Source: CAD feature listing. Evaluate the final solid. Frame: model axes, mm. A direction names the side the tool comes from. Give positions to 0.01 mm unless a question says otherwise; leave off trailing zeros. Loops run counter-clockwise (first coordinate to the right, second up) from the corner with the lowest first, then second, coordinate; pieces in that order, holes last. Notation, with made-up numbers: M 21.25,5.25 L 40.25,5.25 A17 ccw 40.25,33.25 Z; hole C 14.25,32.5 d11. An arc over 180 degrees is marked long. Answer in a Markdown table with one row per item.
```python
from build123d import *

# Parameters (mm, degrees)
SKETCH1_W                      = 40.5
SKETCH1_H                      = 12
F_2_5_2_5_DIAMETER_HOLE1_D     = 2.5
F_2_5_2_5_DIAMETER_HOLE1_DEPTH = 10
F_3_3_3_3_DIAMETER_HOLE1_D     = 3.3
F_3_3_3_3_DIAMETER_HOLE1_DEPTH = 8


with BuildPart() as part:
    # Sketch1 → Revolve1 (revolve)
    with BuildSketch(Plane.XZ, mode=Mode.PRIVATE) as revolve1_sk:
        with Locations((20.25, 6)):
            Rectangle(SKETCH1_W, SKETCH1_H)
    revolve(revolve1_sk.sketch.rotate(Axis((0, 0, 12), (0, 0, -1)), 180), axis=Axis((0, 0, 12), (0, 0, -1)))

    # Ø2.5 (2.5) Diameter Hole1
    with Locations(Plane(origin=(40.5, 0, 6), x_dir=(0, 1, 0), z_dir=(1, 0, 0))):
        with Locations((0, 0)):
            Hole(F_2_5_2_5_DIAMETER_HOLE1_D / 2, depth=F_2_5_2_5_DIAMETER_HOLE1_DEPTH)

    # Ø3.3 (3.3) Diameter Hole1
    with Locations(Plane.XY.offset(12)):
        with Locations((24.748737342, 24.748737342), (-24.748737342, 24.748737342), (24.748737342, -24.748737342), (-24.748737342, -24.748737342)):
            Hole(F_3_3_3_3_DIAMETER_HOLE1_D / 2, depth=F_3_3_3_3_DIAMETER_HOLE1_DEPTH)


solid = part.part
```
1) Pin query (flat end, axial travel): pin 1 Ø3 at (y, z) = (-14.5, 10) entering from -X; pin 2 Ø1 at (x, y) = (25, -25.5) entering from +Z; pin 3 Ø2 at (y, z) = (0, 6) entering from +X. Return the tip coordinate at first contact, or that it passes through.
Reply:
| item | result |
|---|---|
| pin 1 | stops at x = -38.36 |
| pin 2 | stops at z = 4 |
| pin 3 | stops at x = 30.5 |
2) Section A-A, the plane y = 0. Return loops of the section in (x, z), then the cut area to 3 significant figures.
Reply:
| item | result |
|---|---|
| outline | M -40.5,0 L 40.5,0 L 40.5,4.75 L 30.5,4.75 L 30.5,7.25 L 40.5,7.25 L 40.5,12 L -40.5,12 Z |
| area | 947 mm² |
3) Set-up query: faces 4 (the flat face through (-1, 1, 0)), 5 (the cylindrical face through (35.43, 0.27, 4.78)), 6 (the cylindrical face through (-24.39, -26.36, 7.94)). Return all of +Z, -Z, +X, -X, +Y, -Y with unobstructed straight access to the full face (end or side cutting, diameter ignored); none if empty.
Reply:
| item | result |
|---|---|
| face 4 | -Z, +X, -X, +Y, -Y |
| face 5 | +X |
| face 6 | +Z |
4) Section B-B, the plane z = 6. Return loops of the section in (x, y), then the cut area to 3 significant figures.
Reply:
| item | result |
|---|---|
| outline | M 30.5,-1.25 L 30.5,1.25 L 40.48,1.25 A40.5 ccw long 40.48,-1.25 Z; hole C -24.75,-24.75 d3.3; hole C -24.75,24.75 d3.3; hole C 24.75,-24.75 d3.3; hole C 24.75,24.75 d3.3 |
| area | 5,090 mm² |
5) Section C-C, the plane y = -34.5. Return loops of the section in (x, z).
Reply:
| item | result |
|---|---|
| outline | M -21.21,0 L 21.21,0 L 21.21,12 L -21.21,12 Z |
6) Material intervals for L1, parallel to X at y = 24.5, z = 7; L2, parallel to Z at x = 38.5, y = 0; L3, parallel to X at y = -10, z = 5.75, sorted ascending.
Reply:
| item | result |
|---|---|
| L1 | x = -32.25 to -26.38, -23.12 to 23.12, 26.38 to 32.25 |
| L2 | z = 0 to 4.75, 7.25 to 12 |
| L3 | x = -39.25 to 39.25 |
7) Pull-direction query (Z, two-part tool) for faces 1 (the cylindrical face through (-24.39, 23.14, 7.94)), 2 (the flat face through (30.5, 0, 6)), 3 (the flat face through (-25, 25, 4)); classes: released by +Z, released by -Z, zero draft, split by the parting line, or undercut.
Reply:
| item | result |
|---|---|
| face 1 | zero draft |
| face 2 | undercut |
| face 3 | released by +Z |
